The model under review builds one solid part; all positions refer to its coordinate system, in mm. A direction names the side the tool comes from. Give positions to 0.01 mm unless a question says otherwise; leave off trailing zeros. Order: outer loops, then holes, each group sorted by start corner. A loop starts at its lowest first (then second) coordinate and runs counter-clockwise, first axis right, second up. Notation, with made-up numbers: (-38, 74.5) - (-22, 74.5) arc R23 ccw to (-22, 84.5) - close; hole circle Ø5 at (-2, 85). An arc over 180 degrees is marked (long way). Put each result on its own line as item: value.
```python
from build123d import *

# Parameters (mm, degrees)
AUFSATZ_LINEAR_AUSTRAGEN1_DEPTH = 20
SKIZZE2_R                       = 2.05
SKIZZE2_R_2                     = 1.55
SCHNITT_LINEAR_AUSTRAGEN1_DEPTH = 25.5
VERRUNDUNG1_R                   = 5


with BuildPart() as part:
    # Skizze1 → Aufsatz-Linear austragen1 (new body)
    with BuildSketch(Plane(origin=(0, 0, 0), x_dir=(1, 0, 0), z_dir=(0, 1, 0))):
        Polygon((2, -4.5), (-12, -4.5), (-12, -7.5), (12, -7.5), (12, 0), (2, 0), align=None)
    extrude(amount=AUFSATZ_LINEAR_AUSTRAGEN1_DEPTH)

    # Skizze2 → Schnitt-Linear austragen1 (cut, through all)
    with BuildSketch(Plane.XY.offset(7.5)):
        with Locations((-8, 10)):
            Circle(SKIZZE2_R)
        with Locations((7, 15)):
            Circle(SKIZZE2_R_2)
        with Locations((7, 5)):
            Circle(SKIZZE2_R_2)
    extrude(amount=-SCHNITT_LINEAR_AUSTRAGEN1_DEPTH, mode=Mode.SUBTRACT)

    # Verrundung1
    verrundung1_edges = [part.edges().sort_by_distance(p)[0] for p in [
        (-12, 20, 6),
        (12, 20, 3.75),
        (12, 0, 3.75),
        (-12, 0, 6),
    ]]
    fillet(verrundung1_edges, radius=VERRUNDUNG1_R)


solid = part.part
```
(1) The part is to be moulded in two halves that separate along Y. For faces 1 (the flat face through (-12, 10, 6)), 2 (the cylindrical face through (-9.627, 8.753, 6.021)), 3 (the cylindrical face through (10, 1, 4)), 4 (the cylindrical face through (10, 19, 4)), say which applies: pulls with the +Y half, pulls with the -Y half, needs draft (parallel to the pull), parting line crosses it, or undercut.
The answers:
face 1: needs draft
face 2: undercut
face 3: pulls with the -Y half
face 4: pulls with the +Y half
(2) Take a section at B-B, the plane x = -8. Write out the cut boundary in (y, z), then the cut area to 3 significant figures.
The answers:
outline: (0.1, 4.5) - (7.95, 4.5) - (7.95, 7.5) - (0.1, 7.5) - close; (12.05, 4.5) - (19.9, 4.5) - (19.9, 7.5) - (12.05, 7.5) - close
area: 47.1 mm^2
(3) For faces 5 (the cylindrical face through (-10, 1, 6)), 6 (the flat face through (2, 10, 2)), list the 3-axis set-ups (+Z, -Z, +X, -X, +Y, -Y) from which the entire face can be reached by the end or side of a thin tool; tool diameter is ignored.
The answers:
face 5: +Z, -Z, -X, -Y
face 6: -Z, -X, +Y, -Y
(4) Wall thickness on L1, parallel to Z at x = -2, y = 4.75; L2, parallel to X at y = 5.25, z = 1; L3, parallel to X at y = 9.75, z = 4.75: over which ranges is each line inside the solid? List them lowest first.
The answers:
L1: 4.5 to 7.5
L2: 2 to 5.47, 8.53 to 12
L3: -12 to -10.03, -5.97 to 12
(5) Clearance check with flat-ended pins moving along their axes: pin 1 Ø3 at (x, y) = (7, 15) entering from +Z; pin 2 Ø1.5 at (x, y) = (-6, 13) entering from -Z. State where each tip first meets the part, or that it passes through.
The answers:
pin 1: through
pin 2: z = 4.5
(6) Take a section at D-D, the plane y = 12.5. Write out the cut boundary in (x, z).
The answers:
outline: (-12, 4.5) - (2, 4.5) - (2, 0) - (12, 0) - (12, 7.5) - (-12, 7.5) - close
(7) Take a section at A-A, the plane y = 10. Write out the cut boundary in (x, z).
The answers:
outline: (-12, 4.5) - (-10.05, 4.5) - (-10.05, 7.5) - (-12, 7.5) - close; (-5.95, 4.5) - (2, 4.5) - (2, 0) - (12, 0) - (12, 7.5) - (-5.95, 7.5) - close
(8) Take a section at C-C, the plane z = 2.5. Write out the cut boundary in (x, y), then the cut area to 3 significant figures.
The answers:
outline: (2, 0) - (7, 0) arc R5 ccw to (12, 5) - (12, 15) arc R5 ccw to (7, 20) - (2, 20) - close; hole circle Ø3.1 at (7, 5); hole circle Ø3.1 at (7, 15)
area: 174 mm^2
